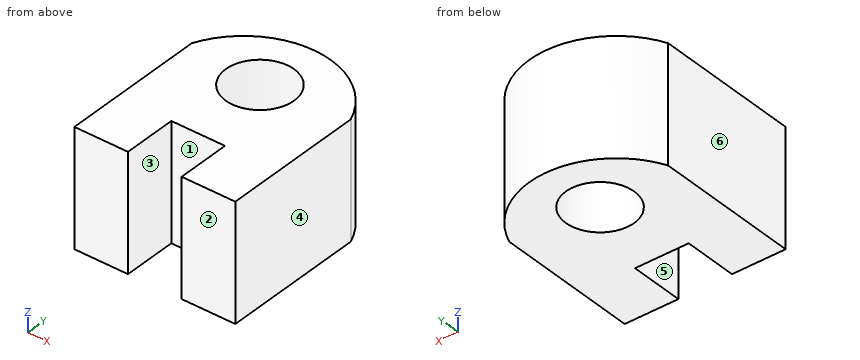
```python
from build123d import *

# Parameters (mm, degrees)
F1_DEPTH = 25.4
F2_DEPTH = 25.4
F3_R     = 14.8837402169
F4_DEPTH = 50.801


with BuildPart() as f1:
    # F0 (on Top) → F1 (new body)
    with BuildSketch(Plane.XY):
        with BuildLine():
            Line((36.7723161906, -34.965459034), (36.7723161906, 27.4711334495))
            ThreePointArc((36.7723161906, 27.4711334495), (2.0053244918, 51.3401081734), (-33.4688444361, 28.5353936383))
            Line((-33.4688444361, 28.5353936383), (-33.4688444361, -34.965459034))
            Line((-33.4688444361, -34.965459034), (-10.0551242272, -34.965459034))
            Line((-10.0551242272, -34.965459034), (-10.0551242272, -11.5517388251))
            Line((-10.0551242272, -11.5517388251), (13.3585959817, -11.5517388251))
            Line((13.3585959817, -11.5517388251), (13.3585959817, -34.965459034))
            Line((13.3585959817, -34.965459034), (36.7723161906, -34.965459034))
        make_face()
    extrude(amount=F1_DEPTH)

    # F2 (add): a face of the model
    f2_faces = [f1.faces().sort_by_distance(p)[0] for p in [
        (1.5994102658, 8.2877292007, 25.4),
    ]]
    extrude(f2_faces, amount=F2_DEPTH)

    # F3 (on face) → F4 (cut, through all)
    with BuildSketch(Plane.XY.offset(50.8)):
        with Locations((0, 23.9132437855)):
            Circle(F3_R)
    extrude(amount=-F4_DEPTH, mode=Mode.SUBTRACT)


solid = f1.part
```
Source: CAD feature listing. Evaluate the final solid. Frame: model axes, mm. Face numbers are marked on the shaded views. A direction names the side the tool comes from. Round coordinates to 2 decimals unless told otherwise and drop trailing zeros. Write each loop counter-clockwise with the first axis right and the second up, starting at its lowest first coordinate (ties: lowest second). Pieces come first, ordered by that corner, then holes. Notation, with made-up numbers: M 38,58 L 69,58 A22 cw 69,86 Z; hole C 28,-19 d2. An arc over 180 degrees is marked long. Use CSV: the item, a comma, the result in double quotes. Start each with the question number.
Q1. Pull-direction query (X, two-part tool) for the marked faces 3, 4, 5 and 6; classes: +X half, -X half, draft (parallel to the pull), parting line (faces both ways), or undercut.
Q2. Cut plane A-A on x = -11.5. Output: boundary loops of the cut face in (y, z), plus the area to 3 significant figures.
Q3. Cut plane C-C on y = 22.5. Output: boundary loops of the cut face in (x, z).
Q4. First-contact query: P1, Ø3, axis at x = 6.5, z = 33, coming from the +Y side; P2, Ø24, axis at x = 0, y = 23.91, coming from the +Z side; P3, Ø1.5, axis at x = 12, z = 34.5, coming from the -Y side. Flat tips, straight axial feed; report the tip coordinate or a pass-through.
Q5. Cut plane B-B on z = 25. Output: boundary loops of the cut face in (x, y), plus the area to 3 significant figures.
Q6. Line query: line 1 (X direction, y = -28.5, z = 36); line 2 (Y direction, x = 0, z = 30); line 3 (X direction, y = 16, z = 10.5). Output: solid intervals per line, ascending. Write a range as from..to.
Q7. Access query for the marked faces 1 and 2. Directions: +Z, -Z, +X, -X, +Y, -Y. A direction counts if a zero-diameter tool reaches every point of the face in a straight line with its end or side. Return the directions, or none.
Q8. Cut plane D-D on x = 24. Output: boundary loops of the cut face in (y, z), plus the area to 3 significant figures.
Results found:
1,face 3,"undercut"
1,face 4,"+X half"
1,face 5,"undercut"
1,face 6,"-X half"
2,outline,"M -34.97,0 L 14.46,0 L 14.46,50.8 L -34.97,50.8 Z; M 33.36,0 L 49.08,0 L 49.08,50.8 L 33.36,50.8 Z"
2,area,"3,310 mm^2"
3,outline,"M -33.47,0 L -14.82,0 L -14.82,50.8 L -33.47,50.8 Z; M 14.82,0 L 36.77,0 L 36.77,50.8 L 14.82,50.8 Z"
4,P1,"y = 51.18"
4,P2,"through"
4,P3,"y = -11.55"
5,outline,"M -33.47,-34.97 L -10.06,-34.97 L -10.06,-11.55 L 13.36,-11.55 L 13.36,-34.97 L 36.77,-34.97 L 36.77,27.47 A38.1 ccw -33.47,28.54 Z; hole C 0,23.91 d29.77"
5,area,"4,360 mm^2"
6,line 1,"-33.47..-10.06, 13.36..36.77"
6,line 2,"-11.55..9.03, 38.8..51.32"
6,line 3,"-33.47..-12.61, 12.61..36.77"
7,face 1,"+Z, -Z, -Y"
7,face 2,"+Z, -Z, +X, -X, -Y"
8,outline,"M -34.97,0 L 43.94,0 L 43.94,50.8 L -34.97,50.8 Z"
8,area,"4,010 mm^2"
